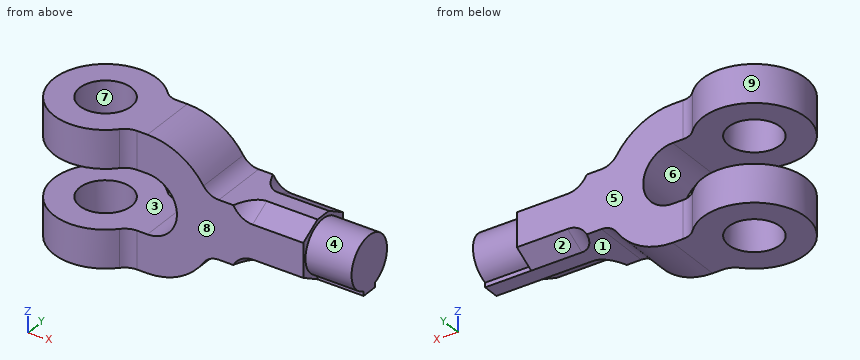
from build123d import *

# Parameters (mm, degrees)
SKETCH2_R                = 56
SKETCH2_R_2              = 28
BOSS_EXTRUDE1_DEPTH      = 41
BOSS_EXTRUDE2_DEPTH      = 31.5
BOSS_EXTRUDE3_REACH      = 173.122
BOSS_EXTRUDE3_END_RADIUS = 56
SKETCH4_W                = 41
SKETCH4_H                = 63
FILLET1_R                = 20
BOSS_EXTRUDE4_REACH      = 317.317
BOSS_EXTRUDE4_END_RADIUS = 73
SKETCH6_W                = 63
SKETCH6_H                = 63
FILLET2_R                = 20
SKETCH7_R                = 28
BOSS_EXTRUDE5_DEPTH      = 50
SKETCH8_R                = 50
CUT_EXTRUDE1_DEPTH       = 80
FILLET3_R                = 25
BOSS_EXTRUDE6_DEPTH      = 50


with BuildPart() as part:
    # Sketch2 → Boss-Extrude1 (new body)
    with BuildSketch(Plane.XY):
        Circle(SKETCH2_R)
        Circle(SKETCH2_R_2, mode=Mode.SUBTRACT)
    extrude(amount=BOSS_EXTRUDE1_DEPTH)


with BuildPart() as body_2:
    # Mirror4: mirrored copy
    add(part.part.mirror(Plane(origin=(0, 0, -32), x_dir=(1, 0, 0), z_dir=(0, 0, -1))))


with BuildPart() as body_3:
    # Sketch3 → Boss-Extrude2 (new, symmetric)
    with BuildSketch(Plane(origin=(0, 0, 0), x_dir=(1, 0, 0), z_dir=(0, 1, 0))):
        with BuildLine():
            Line((66.971041272, 105), (66.971041272, 64))
            ThreePointArc((66.971041272, 64), (98.971041272, 32), (66.971041272, 0))
            Line((66.971041272, 0), (66.971041272, -41))
            ThreePointArc((66.971041272, -41), (139.971041272, 32), (66.971041272, 105))
        make_face()
    extrude(amount=BOSS_EXTRUDE2_DEPTH, both=True)


with BuildPart() as part_1:
    add(part.part)

    add(body_2.part)  # Boss-Extrude3 merges body 2

    add(body_3.part)  # Boss-Extrude3 merges body 3
    # Boss-Extrude3: up to this cylinder (the profile starts outside it)
    boss_extrude3_end = Plane(origin=(0, 0, -32), z_dir=(0, 0, 1)) * Cylinder(BOSS_EXTRUDE3_END_RADIUS, 564.244, mode=Mode.PRIVATE)
    # Sketch4 → Boss-Extrude3 (add, up to the surface)
    with BuildSketch(Plane.ZY.offset(-66.971041272), mode=Mode.PRIVATE) as boss_extrude3_sk1:
        with Locations((20.5, 0)):
            Rectangle(SKETCH4_W, SKETCH4_H)
    boss_extrude3_tool1 = extrude(boss_extrude3_sk1.sketch, amount=BOSS_EXTRUDE3_REACH, mode=Mode.PRIVATE) - boss_extrude3_end
    add(boss_extrude3_tool1.solids().sort_by_distance((66.971041, 0, 20.5))[0])
    # Sketch4 → Boss-Extrude3 (add, up to the surface)
    with BuildSketch(Plane.ZY.offset(-66.971041272), mode=Mode.PRIVATE) as boss_extrude3_sk2:
        with Locations((-84.5, 0)):
            Rectangle(SKETCH4_W, SKETCH4_H)
    boss_extrude3_tool2 = extrude(boss_extrude3_sk2.sketch, amount=BOSS_EXTRUDE3_REACH, mode=Mode.PRIVATE) - boss_extrude3_end
    add(boss_extrude3_tool2.solids().sort_by_distance((66.971041, 0, -84.5))[0])

    # Fillet1
    fillet1_edges = [part_1.edges().sort_by_distance(p)[0] for p in [
        (46.300647944, 31.5, 20.5),
        (46.300647944, -31.5, 20.5),
        (46.300647944, -31.5, -84.5),
        (46.300647944, 31.5, -84.5),
    ]]
    fillet(fillet1_edges, radius=FILLET1_R)

    # Boss-Extrude4: up to this cylinder (the profile starts outside it)
    boss_extrude4_end = Plane(origin=(66.971041272, 0, -32), z_dir=(0, -1, 0)) * Cylinder(BOSS_EXTRUDE4_END_RADIUS, 781.634, mode=Mode.PRIVATE)
    # Sketch6 → Boss-Extrude4 (add, up to the surface)
    with BuildSketch(Plane(origin=(236, 0, 0), x_dir=(0, 0, -1), z_dir=(1, 0, 0)), mode=Mode.PRIVATE) as boss_extrude4_sk1:
        with Locations((32, 0)):
            Rectangle(SKETCH6_W, SKETCH6_H)
    boss_extrude4_tool1 = extrude(boss_extrude4_sk1.sketch, amount=-BOSS_EXTRUDE4_REACH, mode=Mode.PRIVATE) - boss_extrude4_end
    add(boss_extrude4_tool1.solids().sort_by_distance((236, 0, -32))[0])

    # Fillet2
    fillet2_edges = [part_1.edges().sort_by_distance(p)[0] for p in [
        (132.825046465, 0, -0.5),
        (132.825046465, 0, -63.5),
    ]]
    fillet(fillet2_edges, radius=FILLET2_R)

    # Sketch7 → Boss-Extrude5 (add)
    with BuildSketch(Plane(origin=(236, 0, 0), x_dir=(0, 0, -1), z_dir=(1, 0, 0))):
        with Locations((32, 0)):
            Circle(SKETCH7_R)
    extrude(amount=BOSS_EXTRUDE5_DEPTH)

    # Sketch8 → Cut-Extrude1 (cut)
    with BuildSketch(Plane(origin=(236, 0, 0), x_dir=(0, 0, -1), z_dir=(1, 0, 0))):
        with Locations((32, 0)):
            Circle(SKETCH8_R)
        Polygon((68.618122977, 0), (50.309061489, 31.712224737), (13.690938511, 31.712224737), (-4.618122977, 0), (13.690938511, -31.712224737), (50.309061489, -31.712224737), align=None, mode=Mode.SUBTRACT)
    extrude(amount=-CUT_EXTRUDE1_DEPTH, mode=Mode.SUBTRACT)

    # Fillet3
    # the kernel refuses this fillet: 25 mm, written as the material it adds along each edge
    with BuildSketch(Plane(origin=(156, -45.2617387, -94.75), x_dir=(0, 0.5000000000000009, -0.866025403784438), z_dir=(0, 0.8660254037844382, 0.500000000000001))) as fillet3_piece_1_section:
        with BuildLine():
            CenterArc((FILLET3_R, -FILLET3_R), FILLET3_R, 90, 90)
            Line((0, -FILLET3_R), (0, 0))
            Line((0, 0), (FILLET3_R, 0))
        make_face()
    fillet3_piece_1 = extrude(amount=151.136821004, mode=Mode.PRIVATE)
    fillet3_piece_1 = split(fillet3_piece_1, bisect_by=Plane(origin=(163.326286351, 23.024042198, -63.5), z_dir=(0, 0, 1)), keep=Keep.TOP, mode=Mode.PRIVATE)
    fillet3_piece_1 = split(fillet3_piece_1, bisect_by=Plane(origin=(163.326286351, 31.5, -58.606403481), z_dir=(0, -1, 0)), keep=Keep.TOP, mode=Mode.PRIVATE)
    add(fillet3_piece_1)
    with BuildSketch(Plane(origin=(156, -85.626587737, -19.181589498), x_dir=(0, -0.49999999999999484, -0.8660254037844416), z_dir=(0, 0.8660254037844417, -0.49999999999999484))) as fillet3_piece_2_section:
        with BuildLine():
            CenterArc((FILLET3_R, -FILLET3_R), FILLET3_R, 90, 90)
            Line((0, -FILLET3_R), (0, 0))
            Line((0, 0), (FILLET3_R, 0))
        make_face()
    fillet3_piece_2 = extrude(amount=151.136821004, mode=Mode.PRIVATE)
    fillet3_piece_2 = split(fillet3_piece_2, bisect_by=Plane(origin=(163.326286351, -31.5, -58.606403481), z_dir=(0, 1, 0)), keep=Keep.TOP, mode=Mode.PRIVATE)
    fillet3_piece_2 = split(fillet3_piece_2, bisect_by=Plane(origin=(163.326286351, -23.024042198, -63.5), z_dir=(0, 0, 1)), keep=Keep.TOP, mode=Mode.PRIVATE)
    add(fillet3_piece_2)
    with BuildSketch(Plane(origin=(156, 85.626587737, -44.818410502), x_dir=(1, 0, 0), z_dir=(0, -0.8660254037844416, 0.49999999999999506))) as fillet3_piece_3_section:
        with BuildLine():
            CenterArc((FILLET3_R, FILLET3_R), FILLET3_R, 180, 90)
            Line((0, FILLET3_R), (0, 0))
            Line((0, 0), (FILLET3_R, 0))
        make_face()
    fillet3_piece_3 = extrude(amount=151.136821004, mode=Mode.PRIVATE)
    fillet3_piece_3 = split(fillet3_piece_3, bisect_by=Plane(origin=(163.326286352, 23.024042197, -0.5), z_dir=(0, 0, -1)), keep=Keep.TOP, mode=Mode.PRIVATE)
    fillet3_piece_3 = split(fillet3_piece_3, bisect_by=Plane(origin=(163.326286352, 31.5, -5.393596519), z_dir=(0, -1, 0)), keep=Keep.TOP, mode=Mode.PRIVATE)
    add(fillet3_piece_3)
    with BuildSketch(Plane(origin=(156, 45.2617387, 30.75), x_dir=(1, 0, 0), z_dir=(0, -0.8660254037844346, -0.5000000000000071))) as fillet3_piece_4_section:
        with BuildLine():
            CenterArc((FILLET3_R, FILLET3_R), FILLET3_R, 180, 90)
            Line((0, FILLET3_R), (0, 0))
            Line((0, 0), (FILLET3_R, 0))
        make_face()
    fillet3_piece_4 = extrude(amount=151.136821004, mode=Mode.PRIVATE)
    fillet3_piece_4 = split(fillet3_piece_4, bisect_by=Plane(origin=(163.326286352, -31.5, -5.393596519), z_dir=(0, 1, 0)), keep=Keep.TOP, mode=Mode.PRIVATE)
    fillet3_piece_4 = split(fillet3_piece_4, bisect_by=Plane(origin=(163.326286352, -23.024042197, -0.5), z_dir=(0, 0, -1)), keep=Keep.TOP, mode=Mode.PRIVATE)
    add(fillet3_piece_4)

    # Sketch9 → Boss-Extrude6 (add)
    with BuildSketch(Plane(origin=(236, 0, 0), x_dir=(0, 0, -1), z_dir=(1, 0, 0))):
        with BuildLine():
            Line((58.559639523, 8.864849036), (63.5, 8.864849036))
            Line((63.5, 8.864849036), (63.5, -8.864849036))
            Line((63.5, -8.864849036), (58.559639523, -8.864849036))
            ThreePointArc((58.559639523, -8.864849036), (60, 0), (58.559639523, 8.864849036))
        make_face()
    extrude(amount=BOSS_EXTRUDE6_DEPTH)


solid = part_1.part
Model file for the job. Use its own axes, mm. Face numbers are marked on the shaded views. A direction names the side the tool comes from. Coordinates: 2 decimals unless noted, no trailing zeros. Order: outer loops, then holes, each group sorted by start corner. A loop starts at its lowest first (then second) coordinate and runs counter-clockwise, first axis right, second up. Notation, with made-up numbers: (-18.5, -30.75) -> (-1.5, -30.75) arc R6 cw to (-1.5, -25.75) -> close; hole circle Ø9 at (69, -9.75). An arc over 180 degrees is marked (long way). Return JSON: item names as keys, results as strings. Group by question number.
Item 1: Pull direction X, two halves, no side cores. Call the marked faces 6, 7, 8 and 9: pulls with the +X half, pulls with the -X half, needs draft (parallel to the pull), parting line crosses it, or undercut.
Item 2: Saw through at C-C on z = -32. Write the cut outline in (x, y).
Item 3: Flat gauge pins, fed straight in: P1, Ø12, axis at y = -10.5, z = -85.5, coming from the -X side; P2, Ø2.5, axis at x = 259.5, z = -62, coming from the -Y side; P3, Ø8, axis at y = 39.5, z = -58.5, coming from the +X side; P4, Ø8, axis at x = 154.5, y = 21, coming from the +Z side. Where does each tip first touch, or does it go through?
Item 4: Tool access for the marked faces 1, 2, 3, 4 and 5: list every direction of +Z, -Z, +X, -X, +Y, -Y with a clear straight run to the whole face (end or side of a thin tool).
Item 5: Wall check: line 1 along Y through (x, z) = (0, 28); line 2 along Z through (x, y) = (44, -29.5); line 3 along X through (y, z) = (2, -79.5). Give the ranges that are in metal, low to high. Write a range as [from, to].
Item 6: Saw through at D-D on x = 171.5. Write the cut outline in (y, z).
Item 7: Saw through at B-B on y = 0. Write the cut outline in (x, z), then the cut area to 3 significant figures.
Item 8: Saw through at A-A on x = 0. Write the cut outline in (y, z), then the cut area to 3 significant figures.
Values found:
{
 "1": {"face 6": "pulls with the -X half", "face 7": "undercut", "face 8": "needs draft", "face 9": "parting line crosses it"},
 "2": {"outline": "(98.97, -31.5) -> (236, -31.5) -> (236, -28) -> (286, -28) -> (286, 28) -> (236, 28) -> (236, 31.5) -> (98.97, 31.5) -> close"},
 "3": {"P1": "stops at x = -55.82", "P2": "stops at y = -8.86", "P3": "passes through", "P4": "stops at z = -0.5"},
 "4": {"face 1": "-Z, +X, +Y, -Y", "face 2": "-Z, +X, +Y", "face 3": "-X, +Y, -Y", "face 4": "+X", "face 5": "+Z, -Z, +X, +Y"},
 "5": {"line 1": "y = [-56, -28], [28, 56]", "line 2": "z = [-105, -64], [0, 41]", "line 3": "x = [-55.96, -27.93], [27.93, 122.4]"},
 "6": {"outline": "(-31.5, -52.6) -> (-12.62, -63.5) -> (12.62, -63.5) -> (31.5, -52.6) -> (31.5, -11.4) -> (12.62, -0.5) -> (-12.62, -0.5) -> (-31.5, -11.4) -> close"},
 "7": {"outline": "(-56, -105) -> (-28, -105) -> (-28, -64) -> (-56, -64) -> close; (-56, 0) -> (-28, 0) -> (-28, 41) -> (-56, 41) -> close; (28, -105) -> (66.97, -105) arc R73 ccw to (127.76, -72.42) arc R20 cw to (144.41, -63.5) -> (286, -63.5) -> (286, -4) -> (236, -4) -> (236, -0.5) -> (144.41, -0.5) arc R20 cw to (127.76, 8.42) arc R73 ccw to (66.97, 41) -> (28, 41) -> (28, 0) -> (66.97, 0) arc R32 cw to (66.97, -64) -> (28, -64) -> close", "area": "21,500 mm2"},
 "8": {"outline": "(-56, -105) -> (-28, -105) -> (-28, -64) -> (-56, -64) -> close; (-56, 0) -> (-28, 0) -> (-28, 41) -> (-56, 41) -> close; (28, -105) -> (56, -105) -> (56, -64) -> (28, -64) -> close; (28, 0) -> (56, 0) -> (56, 41) -> (28, 41) -> close", "area": "4,590 mm2"}
}
